The drawing under review shows one solid part. Ordinate dimensions are in mm from its lowest x, y, z. Give positions to 0.01 mm unless a question says otherwise; leave off trailing zeros. Order: outer loops, then holes, each group sorted by start corner. A loop starts at its lowest first (then second) coordinate and runs counter-clockwise, first axis right, second up. Notation, with made-up numbers: (-19, 25.5) - (37, 25.5) arc R33 cw to (37, 64.5) - close; hole circle Ø9 at (81, 23). An arc over 180 degrees is marked (long way). Write item = value, one per line. Start each with the question number.
1. Wall thickness on probe 1 along Y at (x, z) = (30, 2.6): over which ranges is the line inside the solid? List them lowest first.
2. For P1, Ø7, axis at x = 30, y = 152, coming from the +Z side, flat-tipped, find the tip position at first contact; note if it passes through.
3. We need section A-A, the plane x = 30. Give the boundary of the cut face in (y, z).
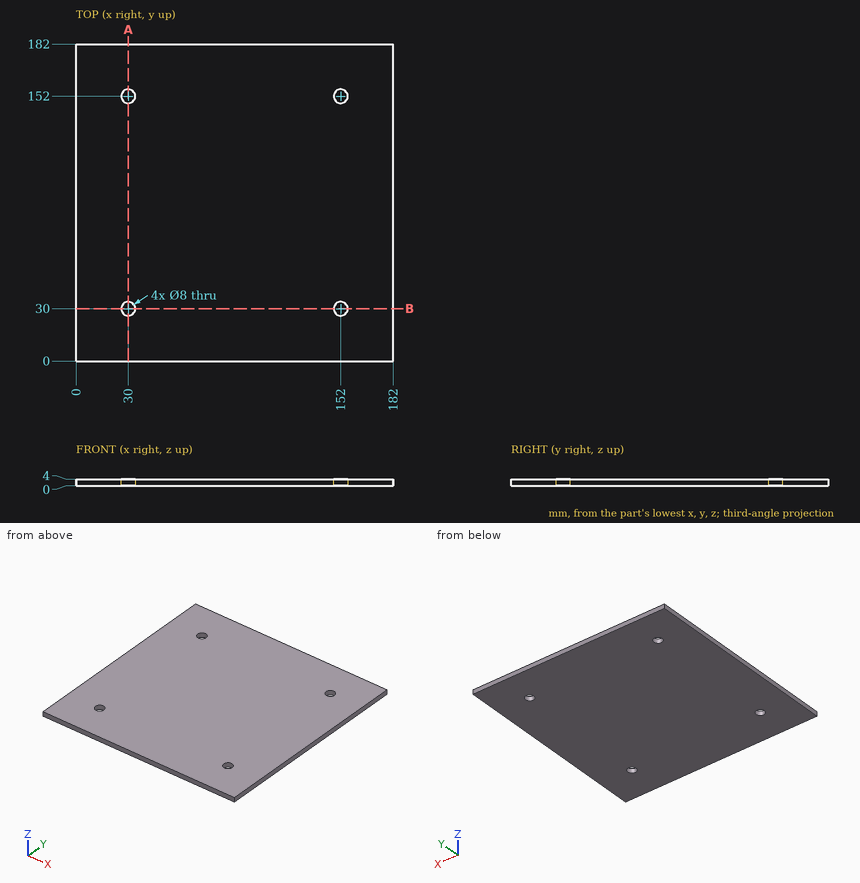
Model answer:
q1.probe_1 = 0 to 26, 34 to 148, 156 to 182
q2.P1 = through
q3.outline = (0, 0) - (26, 0) - (26, 4) - (0, 4) - close; (34, 0) - (148, 0) - (148, 4) - (34, 4) - close; (156, 0) - (182, 0) - (182, 4) - (156, 4) - close
